For this review, take the finished solid that the model builds, in its own axes (mm). A direction names the side the tool comes from. Give positions to 0.01 mm unless a question says otherwise; leave off trailing zeros. Loops run counter-clockwise (first coordinate to the right, second up) from the corner with the lowest first, then second, coordinate; pieces in that order, holes last. Notation, with made-up numbers: (-17, 85.25) - (-1, 85.25) arc R14 cw to (-1, 92.25) - close; hole circle Ø2 at (20, 14). An arc over 180 degrees is marked (long way). Use CSV: the item, a comma, the result in double quotes. Start each with the question number.
1. Take a section at A-A on z = 5. Give the boundary of the cut face in (x, y).
2. Take a section at C-C on x = 6.75. Give the boundary of the cut face in (y, z), plus the area to 3 significant figures.
3. Take a section at B-B on y = 1.25. Give the boundary of the cut face in (x, z).
4. Take a section at D-D on z = 0.75. Give the boundary of the cut face in (x, y).
5. Mouldability with a two-part tool opening along X and no side actions: class faces 1 (the cylindrical face through (6.9, 7.2, 4.9)), 2 (the flat face through (7, 3, 0)), 3 (the flat face through (7, 4, 5)) as pulls with the +X half, pulls with the -X half, needs draft (parallel to the pull), parting line crosses it, or undercut.
6. For pin 1 (2 mm diameter, centred on x = 7.5, z = 6, fed in from -Y), flat-tipped, find the tip position at first contact; note if it passes through.
7. Wall thickness on line 1 (X direction, y = 3, z = 5); line 2 (X direction, y = 3, z = 8.25); line 3 (Y direction, x = 2.5, z = 8.25): over which ranges is each line inside the solid? List them lowest first.
8. For faces 4 (the flat face through (7, 3, 10)), 5 (the cylindrical face through (9.786, 2.226, 3.065)), list the 3-axis set-ups (+Z, -Z, +X, -X, +Y, -Y) from which the entire face can be reached by the end or side of a thin tool; tool diameter is ignored.
```python
from build123d import *

# Parameters (mm, degrees)
BOSS_EXTRUDE1_DEPTH = 10
SKETCH2_R           = 3.6
CUT_EXTRUDE1_DEPTH  = 4
CHAMFER1_SIZE       = 0.5


with BuildPart() as part:
    # Sketch1 → Boss-Extrude1 (new body)
    with BuildSketch(Plane.XY):
        with BuildLine():
            Line((0, 0), (13.5, 0))
            Line((13.5, 0), (13.5, 2))
            ThreePointArc((13.5, 2), (6.75, 7.2), (0, 2))
            Line((0, 2), (0, 0))
        make_face()
    extrude(amount=BOSS_EXTRUDE1_DEPTH)

    # Sketch2 → Cut-Extrude1 (cut)
    with BuildSketch(Plane.XZ):
        with Locations(Location((6.75, 5, 0), (0, 0, 270))):
            Circle(SKETCH2_R)
    extrude(amount=-CUT_EXTRUDE1_DEPTH, mode=Mode.SUBTRACT)

    # Chamfer1
    chamfer1_edges = [part.edges().sort_by_distance(p)[0] for p in [
        (6.75, 0, 8.6),
        (6.75, 0, 0),
        (6.75, 0, 10),
        (13.5, 0, 5),
        (0, 0, 5),
    ]]
    chamfer(chamfer1_edges, length=CHAMFER1_SIZE)


solid = part.part
```
Check result:
1,outline,"(0, 0.5) - (0.5, 0) - (2.65, 0) - (3.15, 0.5) - (3.15, 4) - (10.35, 4) - (10.35, 0.5) - (10.85, 0) - (13, 0) - (13.5, 0.5) - (13.5, 2) arc R6.98 ccw to (0, 2) - close"
2,outline,"(0, 0.5) - (0.5, 0) - (7.2, 0) - (7.2, 10) - (0.5, 10) - (0, 9.5) - (0, 9.1) - (0.5, 8.6) - (4, 8.6) - (4, 1.4) - (0.5, 1.4) - (0, 0.9) - close"
2,area,"42.7 mm²"
3,outline,"(0, 0) - (13.5, 0) - (13.5, 10) - (0, 10) - close; hole circle Ø7.2 at (6.75, 5)"
4,outline,"(0, 0.5) - (0.5, 0) - (13, 0) - (13.5, 0.5) - (13.5, 2) arc R6.98 ccw to (0, 2) - close"
5,face 1,"parting line crosses it"
5,face 2,"needs draft"
5,face 3,"undercut"
6,pin 1,"stops at y = 4"
7,line 1,"x = 0.35 to 3.15, 10.35 to 13.15"
7,line 2,"x = 0.35 to 5.2, 8.3 to 13.15"
7,line 3,"y = 0 to 5.76"
8,face 4,"+Z, +X, -X, +Y, -Y"
8,face 5,"-Y"
